from build123d import *

# Parameters (mm, degrees)
ESQUISSE1_W                      = 83
ESQUISSE1_H                      = 6
BOSS_EXTRU_1_DEPTH               = 5
ENL_V_MAT_EXTRU_1_DEPTH          = 5
CONG_1_R                         = 0.2
R_P_TITION_LIN_AIRE4_COUNT       = 9
R_P_TITION_LIN_AIRE4_PITCH       = 9
CONG_1_OF_R_P_TITION_LIN_AIRE4_R = 0.2
CONG_2_R                         = 0.2
ESQUISSE3_W                      = 10
ESQUISSE3_H                      = 6
BOSS_EXTRU_2_DEPTH               = 3
ESQUISSE4_W                      = 10
ESQUISSE4_H                      = 3
BOSS_EXTRU_3_DEPTH               = 14
ESQUISSE5_R                      = 1.9
ENL_V_MAT_EXTRU_2_DEPTH          = 15
CONG_3_R                         = 1
CHANFREIN1_SIZE                  = 0.5
ESQUISSE6_W                      = 1.5
ESQUISSE6_H                      = 1.9
BOSS_EXTRU_4_DEPTH               = 4
CHANFREIN2_SIZE                  = 2


with BuildPart() as part:
    # Esquisse1 → Boss.-Extru.1 (new body)
    with BuildSketch(Plane(origin=(0, 0, 0), x_dir=(0, 0, -1), z_dir=(1, 0, 0))):
        Rectangle(ESQUISSE1_W, ESQUISSE1_H)
    extrude(amount=BOSS_EXTRU_1_DEPTH)

    # Esquisse2 → Enlèv. mat.-Extru.1 (cut)
    with BuildSketch(Plane(origin=(5, 0, 0), x_dir=(0, 0, -1), z_dir=(1, 0, 0))):
        Polygon((-38.5, 3), (-41.5, 3), (-40, 1), align=None)
        Polygon((-35.5, 3), (-38.5, 3), (-37, 1), align=None)
        Polygon((-32.5, 3), (-35.5, 3), (-34, 1), align=None)
    enl_v_mat_extru_1 = extrude(amount=-ENL_V_MAT_EXTRU_1_DEPTH, mode=Mode.SUBTRACT)

    # Congé1
    cong_1_edges = [part.edges().sort_by_distance(p)[0] for p in [
        (2.5, 1, 40),
        (2.5, 3, 38.5),
        (2.5, 1, 34),
        (2.5, 1, 37),
        (2.5, 3, 35.5),
    ]]
    fillet(cong_1_edges, radius=CONG_1_R)

    # Répétition linéaire4: Enlèv. mat.-Extru.1 ×9
    with Locations(*[(0, 0, -i * R_P_TITION_LIN_AIRE4_PITCH) for i in range(1, R_P_TITION_LIN_AIRE4_COUNT)]):
        add(enl_v_mat_extru_1, mode=Mode.SUBTRACT)

    # Congé1 of Répétition linéaire4
    cong_1_of_r_p_tition_lin_aire4_edges = [part.edges().sort_by_distance(p)[0] for p in [
        (2.5, 1, 31),
        (2.5, 3, 29.5),
        (2.5, 1, 25),
        (2.5, 1, 28),
        (2.5, 3, 26.5),
        (2.5, 1, 22),
        (2.5, 3, 20.5),
        (2.5, 1, 16),
        (2.5, 1, 19),
        (2.5, 3, 17.5),
        (2.5, 1, 13),
        (2.5, 3, 11.5),
        (2.5, 1, 7),
        (2.5, 1, 10),
        (2.5, 3, 8.5),
        (2.5, 1, 4),
        (2.5, 3, 2.5),
        (2.5, 1, -2),
        (2.5, 1, 1),
        (2.5, 3, -0.5),
        (2.5, 1, -5),
        (2.5, 3, -6.5),
        (2.5, 1, -11),
        (2.5, 1, -8),
        (2.5, 3, -9.5),
        (2.5, 1, -14),
        (2.5, 3, -15.5),
        (2.5, 1, -20),
        (2.5, 1, -17),
        (2.5, 3, -18.5),
        (2.5, 1, -23),
        (2.5, 3, -24.5),
        (2.5, 1, -29),
        (2.5, 1, -26),
        (2.5, 3, -27.5),
        (2.5, 1, -32),
        (2.5, 3, -33.5),
        (2.5, 1, -38),
        (2.5, 1, -35),
        (2.5, 3, -36.5),
    ]]
    fillet(cong_1_of_r_p_tition_lin_aire4_edges, radius=CONG_1_OF_R_P_TITION_LIN_AIRE4_R)

    # Congé2
    cong_2_edges = [part.edges().sort_by_distance(p)[0] for p in [
        (2.5, 3, 23.5),
        (2.5, 3, 5.5),
        (2.5, 3, -12.5),
        (2.5, 3, -30.5),
        (2.5, 3, 14.5),
        (2.5, 3, -3.5),
        (2.5, 3, 32.5),
        (2.5, 3, -21.5),
        (2.5, 3, -39.5),
        (2.5, 3, 41.5),
    ]]
    fillet(cong_2_edges, radius=CONG_2_R)

    # Esquisse3 → Boss.-Extru.2 (add)
    with BuildSketch(Plane(origin=(0, 0, -41.5), x_dir=(-1, 0, 0), z_dir=(0, 0, -1))):
        with Locations((-2.5, 0)):
            Rectangle(ESQUISSE3_W, ESQUISSE3_H)
    extrude(amount=BOSS_EXTRU_2_DEPTH)

    # Esquisse4 → Boss.-Extru.3 (add)
    with BuildSketch(Plane(origin=(0, 3, 0), x_dir=(1, 0, 0), z_dir=(0, 1, 0))):
        with Locations((2.5, 43)):
            Rectangle(ESQUISSE4_W, ESQUISSE4_H)
    extrude(amount=BOSS_EXTRU_3_DEPTH)

    # Esquisse5 → Enlèv. mat.-Extru.2 (cut)
    with BuildSketch(Plane(origin=(0, 0, -44.5), x_dir=(-1, 0, 0), z_dir=(0, 0, -1))):
        with Locations((-2.5, 9.5)):
            Circle(ESQUISSE5_R)
    extrude(amount=-ENL_V_MAT_EXTRU_2_DEPTH, mode=Mode.SUBTRACT)

    # Congé3
    cong_3_edges = [part.edges().sort_by_distance(p)[0] for p in [
        (-2.5, 17, -43),
        (7.5, 17, -43),
    ]]
    fillet(cong_3_edges, radius=CONG_3_R)

    # Chanfrein1
    chanfrein1_edges = [part.edges().sort_by_distance(p)[0] for p in [
        (4.4, 9.5, -41.5),
    ]]
    chamfer(chanfrein1_edges, length=CHANFREIN1_SIZE)

    # Esquisse6 → Boss.-Extru.4 (add)
    with BuildSketch(Plane(origin=(0, 3, 0), x_dir=(1, 0, 0), z_dir=(0, 1, 0))):
        with Locations((2.5, 40.55)):
            Rectangle(ESQUISSE6_W, ESQUISSE6_H)
    extrude(amount=BOSS_EXTRU_4_DEPTH)

    # Chanfrein2
    # the kernel refuses this chamfer: 2 mm, written as the material it takes off along each edge
    with BuildSketch(Plane(origin=(-3.393365976, 7, -39.6), x_dir=(0, 0.02749587661058651, -0.9996219169112968), z_dir=(1, 0, 0))) as chanfrein2_piece_1_section:
        Polygon((CHANFREIN2_SIZE * 0.999621916911, -CHANFREIN2_SIZE * 0.0274958766106), (-CHANFREIN2_SIZE * 0.0274958766106, -CHANFREIN2_SIZE * 0.999621916911), (0, 0), align=None)
    chanfrein2_piece_1 = extrude(amount=11.786731952, mode=Mode.PRIVATE)
    chanfrein2_piece_1 = split(chanfrein2_piece_1, bisect_by=Plane(origin=(2.5, 6.33491081, -41.5), z_dir=(0, 0, 1)), keep=Keep.TOP, mode=Mode.PRIVATE)
    add(chanfrein2_piece_1, mode=Mode.SUBTRACT)


solid = part.part
Geometry check sheet. Reference: the model listing, model coordinates, mm. A direction names the side the tool comes from. Round coordinates to 2 decimals unless told otherwise and drop trailing zeros. Write each loop counter-clockwise with the first axis right and the second up, starting at its lowest first coordinate (ties: lowest second). Pieces come first, ordered by that corner, then holes. Notation, with made-up numbers: (-11.5, -23.5) -> (22.5, -23.5) arc R27 ccw to (22.5, -1.5) -> close; hole circle Ø3 at (-14, -34.5). An arc over 180 degrees is marked (long way). One line per item, written item: value. Start each with the question number.
(1) Cross-section at A-A, the plane y = 9.5. Record the cut outline in (x, z), and give its area (4 significant figures).
(2) Cross-section at C-C, the plane y = 13.5. Record the cut outline in (x, z).
(3) Cross-section at B-B, the plane y = 0. Record the cut outline in (x, z), and give its area (3 significant figures).
(4) Access from +Z, -Z, +X, -X, +Y, -Y to the whole of each face (thin tool, end or side, straight path). Record for faces 4 (the flat face through (3.25, 4, -41)), 5 (the flat face through (2.535, 2.011, -25.242)), 6 (the flat face through (-2.5, 6, -43)).
(5) Scan lines: line 1 (Y direction, x = 2.5, z = -43.6); line 2 (Z direction, x = 4.5, y = 5.25); line 3 (Y direction, x = 0.75, z = 33). Record each from-to range of solid material in increasing order. Write a range as [from, to].
(6) Go/stop test with flat-tipped pins: pin 1 Ø1.9 at (x, z) = (1, -40.5) entering from +Y; pin 2 Ø1 at (x, y) = (3.5, 12.5) entering from +Z; pin 3 Ø6.5 at (y, z) = (1.5, 4) entering from -X; pin 4 Ø2.5 at (x, y) = (2.5, 9.5) entering from +Z. Record where each tip stops, or that it passes through.
(7) Draft check along Z on faces 1 (the flat face through (2.535, 2.011, 22.758)), 2 (the flat face through (2, 0, 41.5)), 3 (the flat face through (1, 3, -41)). Enter one of: +Z half, -Z half, draft (parallel to the pull), parting line (faces both ways), or undercut.
Answer:
1. outline: (-2.5, -44.5) -> (0.6, -44.5) -> (0.6, -42) -> (0.1, -41.5) -> (-2.5, -41.5) -> close; (4.4, -44.5) -> (7.5, -44.5) -> (7.5, -41.5) -> (4.9, -41.5) -> (4.4, -42) -> close
1. area: 18.35 mm²
2. outline: (-2.5, -44.5) -> (7.5, -44.5) -> (7.5, -41.5) -> (-2.5, -41.5) -> close
3. outline: (-2.5, -44.5) -> (7.5, -44.5) -> (7.5, -41.5) -> (5, -41.5) -> (5, 41.5) -> (0, 41.5) -> (0, -41.5) -> (-2.5, -41.5) -> close
3. area: 445 mm²
4. face 4: +Z, +X, +Y
4. face 5: +X, -X, +Y
4. face 6: +Z, -Z, -X, +Y, -Y
5. line 1: [-3, 7.6], [11.4, 17]
5. line 2: [-44.5, -41.5]
5. line 3: [-3, 2.33]
6. pin 1: y = 6.48
6. pin 2: z = -41.5
6. pin 3: x = 0
6. pin 4: through
7. face 1: undercut
7. face 2: +Z half
7. face 3: draft
